Geometry check sheet. Reference: drawing and pictorial views, mm from the part's lowest x, y, z. A direction names the side the tool comes from. Round coordinates to 2 decimals unless told otherwise and drop trailing zeros. Loops run counter-clockwise (first coordinate to the right, second up) from the corner with the lowest first, then second, coordinate; pieces in that order, holes last. Notation, with made-up numbers: (19, 68) -> (42, 68) arc R17 cw to (42, 89) -> close; hole circle Ø11 at (80, 63). An arc over 180 degrees is marked (long way). Use one line per item in the form item = value.
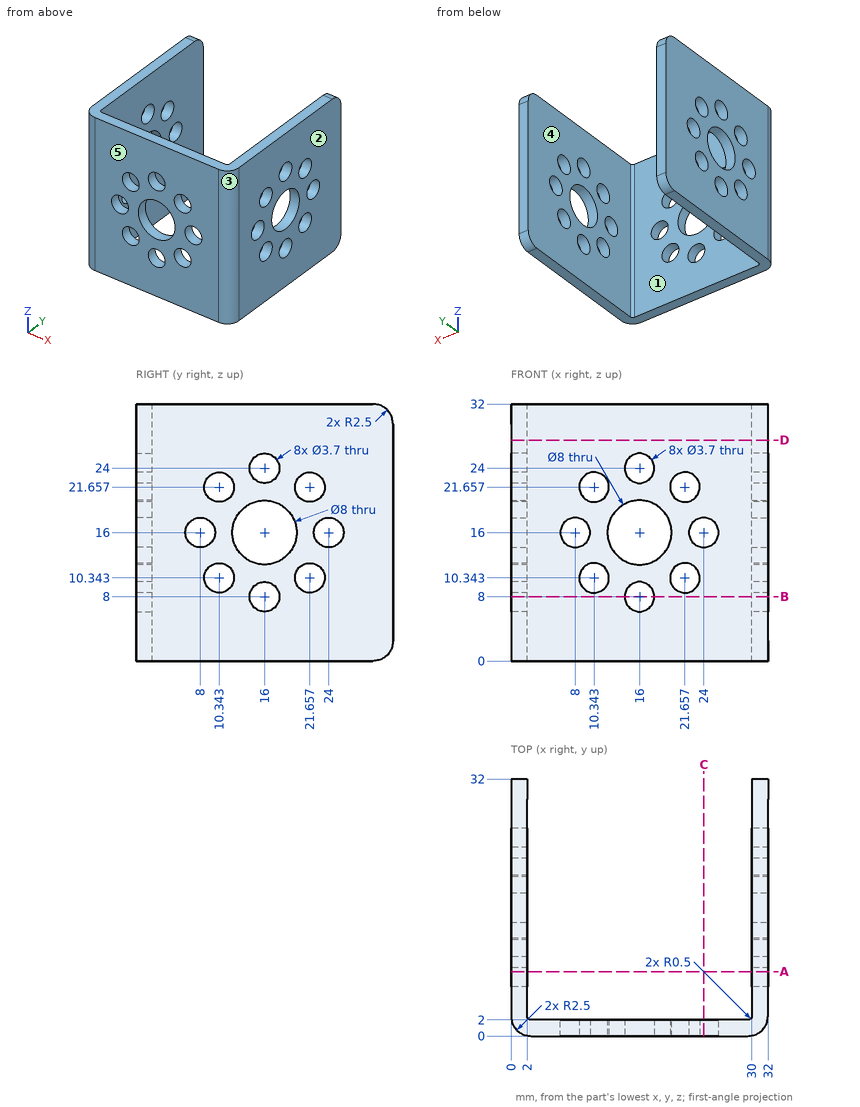
1. Gauge pin test, flat ends, axial feed: pin 1 (10 mm diameter, centred on x = 9.5, z = 7, fed in from +Y); pin 2 (3 mm diameter, centred on y = 10.34, z = 10.34, fed in from +X). Record the tip position at first contact, or that the pin passes through.
Return value:
pin_1 = 2
pin_2 = through
2. Material ranges on line 1 along X through (y, z) = (8, 8); line 2 along Y through (x, z) = (26.5, 15); line 3 along X through (y, z) = (1.5, 26.5), recorded low to high.
Return value:
line_1 = 0 to 2, 30 to 32
line_2 = 0 to 2
line_3 = 0.21 to 31.79
3. Tool access check on the marked faces 1 and 2. Record the directions out of +Z, -Z, +X, -X, +Y, -Y that give a thin tool (end or side, any length) a straight path to the whole face; none if there is none.
Return value:
face_1 = +Z, -Z, +Y
face_2 = +Z, -Z, +X, +Y, -Y
4. Section check C-C (x = 24). Record the boundary of the cut face in (y, z), then the cut area to 3 significant figures.
Return value:
outline = (0, 0) -> (2, 0) -> (2, 14.15) -> (0, 14.15) -> close; (0, 17.85) -> (2, 17.85) -> (2, 32) -> (0, 32) -> close
area = 56.6 mm2
5. Section check B-B (z = 8). Record the boundary of the cut face in (x, y).
Return value:
outline = (0, 2.5) arc R2.5 ccw to (2.5, 0) -> (14.15, 0) -> (14.15, 2) -> (2.5, 2) arc R0.5 cw to (2, 2.5) -> (2, 14.15) -> (0, 14.15) -> close; (0, 17.85) -> (2, 17.85) -> (2, 32) -> (0, 32) -> close; (17.85, 0) -> (29.5, 0) arc R2.5 ccw to (32, 2.5) -> (32, 14.15) -> (30, 14.15) -> (30, 2.5) arc R0.5 cw to (29.5, 2) -> (17.85, 2) -> close; (30, 17.85) -> (32, 17.85) -> (32, 32) -> (30, 32) -> close
6. Mould release check, pull along X, two halves, no side actions. Record for the marked faces 3, 4 and 5: released by +X, released by -X, zero draft, split by the parting line, or undercut.
Return value:
face_3 = released by +X
face_4 = undercut
face_5 = zero draft
7. Section check A-A (y = 8). Record the boundary of the cut face in (x, z).
Return value:
outline = (0, 0) -> (2, 0) -> (2, 14.15) -> (0, 14.15) -> close; (0, 17.85) -> (2, 17.85) -> (2, 32) -> (0, 32) -> close; (30, 0) -> (32, 0) -> (32, 14.15) -> (30, 14.15) -> close; (30, 17.85) -> (32, 17.85) -> (32, 32) -> (30, 32) -> close
8. Section check D-D (z = 27.5). Record the boundary of the cut face in (x, y), then the cut area to 3 significant figures.
Return value:
outline = (0, 2.5) arc R2.5 ccw to (2.5, 0) -> (29.5, 0) arc R2.5 ccw to (32, 2.5) -> (32, 32) -> (30, 32) -> (30, 2.5) arc R0.5 cw to (29.5, 2) -> (2.5, 2) arc R0.5 cw to (2, 2.5) -> (2, 32) -> (0, 32) -> close
area = 181 mm2
